CAD build for the part. Positions are in the model's coordinates, mm. Face numbers are marked on the shaded views. Give positions to 0.01 mm unless a question says otherwise; leave off trailing zeros. Order: outer loops, then holes, each group sorted by start corner. A loop starts at its lowest first (then second) coordinate and runs counter-clockwise, first axis right, second up.
Item 1: Band-saw the part on B-B on y = -1.75. Give the cut face in (x, z).
Item 2: Two-plate mould, pull along X, no slides. Class the marked faces 1, 2, 3 and 4: released by +X, released by -X, zero draft, split by the parting line, or undercut.
Item 3: Wall check: L1, parallel to X at y = -1.5, z = 0.1; L2, parallel to X at y = 2.5, z = 0.2; L3, parallel to Y at x = 1.5, z = 0.3. Give the ranges that are in metal, low to high.
Item 4: Band-saw the part on C-C on x = -1.75. Give the cut face in (y, z), plus the area to 3 significant figures.
Item 5: Band-saw the part on A-A on z = -0.2. Give the cut face in (x, y), plus the area to 3 significant figures.
Item 6: Band-saw the part on D-D on x = 0. Give the cut face in (y, z), plus the area to 3 significant figures.
Item 7: Flat gauge pin, fed straight in: P1, Ø1, axis at x = 2, y = 1.5, coming from the +Z side. Where does the tip first touch, or does it go through?
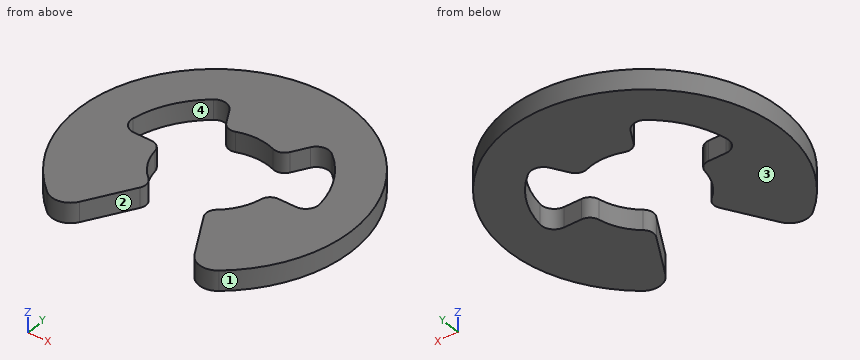
Autodesk Inventor part; units mm, degrees
ref_plane "RR_XY" through (0, 0, 0) normal (0, 0, 1) x (1, 0, 0)
ref_plane "RR_YZ" through (0, 0, 0) normal (1, 0, 0) x (0, 1, 0)
ref_plane "RR_ZX" through (0, 0, 0) normal (0, 1, 0) x (0, 0, 1)
sketch "Sketch_1" plane through (0, 0, 0) normal (0, 0, 1) x (1, 0, 0)
  arc A0 (3.0189, -3.6834) -> (-3.0189, -3.6834) centre (0, 0) ccw
  arc A1 (-3.0189, -3.6834) -> (-2.0217, -3.5017) centre (-2.5975, -3.1692) ccw
  line L0 (-2.0217, -3.5017) -> (-1.1157, -1.9325)
  arc A2 (-1.1157, -1.9325) -> (-1.202, -1.4533) centre (-1.4424, -1.7439) ccw
  arc A3 (-1.8596, -0.3143) -> (-1.202, -1.4533) centre (0, 0) ccw
  arc A4 (-1.8596, -0.3143) -> (-2.2315, 0) centre (-2.2315, -0.3772) ccw
  line L1 (-2.2315, 0) -> (-2.8467, 0)
  arc A5 (-3.2846, 0.5114) -> (-2.8467, 0) centre (-2.8467, 0.4432) ccw
  arc A6 (-2.0852, 2.5889) -> (-3.2846, 0.5114) centre (0, 0) ccw
  arc A7 (-1.4233, 2.4653) -> (-2.0852, 2.5889) centre (-1.8072, 2.2437) ccw
  line L2 (-1.4233, 2.4653) -> (-1.1157, 1.9325)
  arc A8 (-1.1157, 1.9325) -> (-0.6576, 1.7676) centre (-0.7891, 2.1211) ccw
  arc A9 (0.6576, 1.7676) -> (-0.6576, 1.7676) centre (0, 0) ccw
  arc A10 (0.6576, 1.7676) -> (1.1157, 1.9325) centre (0.7891, 2.1211) ccw
  line L3 (1.1157, 1.9325) -> (1.4233, 2.4653)
  arc A11 (2.0852, 2.5889) -> (1.4233, 2.4653) centre (1.8072, 2.2437) ccw
  arc A12 (3.2846, 0.5114) -> (2.0852, 2.5889) centre (0, 0) ccw
  arc A13 (2.8467, 0) -> (3.2846, 0.5114) centre (2.8467, 0.4432) ccw
  line L4 (2.8467, 0) -> (2.2315, 0)
  arc A14 (2.2315, 0) -> (1.8596, -0.3143) centre (2.2315, -0.3772) ccw
  arc A15 (1.202, -1.4533) -> (1.8596, -0.3143) centre (0, 0) ccw
  arc A16 (1.202, -1.4533) -> (1.1157, -1.9325) centre (1.4424, -1.7439) ccw
  line L5 (1.1157, -1.9325) -> (2.0217, -3.5017)
  arc A17 (2.0217, -3.5017) -> (3.0189, -3.6834) centre (2.5975, -3.1692) ccw
extrude "Extrusion1" add sketch "Sketch_1" along normal mid plane 0.6985
ref_plane "RR_XY" through (0, 0, 0) normal (0, 0, 1) x (1, 0, 0)
ref_plane "RR_YZ" through (0, 0, 0) normal (1, 0, 0) x (0, 1, 0)
ref_plane "RR_ZX" through (0, 0, 0) normal (0, 1, 0) x (0, 0, 1)
properties part number "D-5406"
The answers:
1. outline: (-4.43, -0.35) - (-1.07, -0.35) - (-1.07, 0.35) - (-4.43, 0.35) - close; (1.07, -0.35) - (4.43, -0.35) - (4.43, 0.35) - (1.07, 0.35) - close
2. face 1: split by the parting line
2. face 2: undercut
2. face 3: zero draft
2. face 4: undercut
3. L1: x = -4.52 to -1.15, 1.15 to 4.52
3. L2: x = -4.05 to -2.19, -1.45 to 1.45, 2.19 to 4.05
3. L3: y = -2.6 to -1.14, 2.56 to 4.52
4. outline: (-3.03, -0.35) - (-0.7, -0.35) - (-0.7, 0.35) - (-3.03, 0.35) - close; (2.68, -0.35) - (4.43, -0.35) - (4.43, 0.35) - (2.68, 0.35) - close
4. area: 2.85 mm2
5. outline: (-3.28, 0.51) arc R3.32 cw to (-2.09, 2.59) arc R0.44 cw to (-1.42, 2.47) - (-1.12, 1.93) arc R0.38 ccw to (-0.66, 1.77) arc R1.89 cw to (0.66, 1.77) arc R0.38 ccw to (1.12, 1.93) - (1.42, 2.47) arc R0.44 cw to (2.09, 2.59) arc R3.32 cw to (3.28, 0.51) arc R0.44 cw to (2.85, 0) - (2.23, 0) arc R0.38 ccw to (1.86, -0.31) arc R1.89 cw to (1.2, -1.45) arc R0.38 ccw to (1.12, -1.93) - (2.02, -3.5) arc R0.66 ccw to (3.02, -3.68) arc R4.76 ccw (long way) to (-3.02, -3.68) arc R0.66 ccw to (-2.02, -3.5) - (-1.12, -1.93) arc R0.38 ccw to (-1.2, -1.45) arc R1.89 cw to (-1.86, -0.31) arc R0.38 ccw to (-2.23, 0) - (-2.85, 0) arc R0.44 cw to start
5. area: 42.1 mm2
6. outline: (1.89, -0.35) - (4.76, -0.35) - (4.76, 0.35) - (1.89, 0.35) - close
6. area: 2.01 mm2
7. P1: passes through
